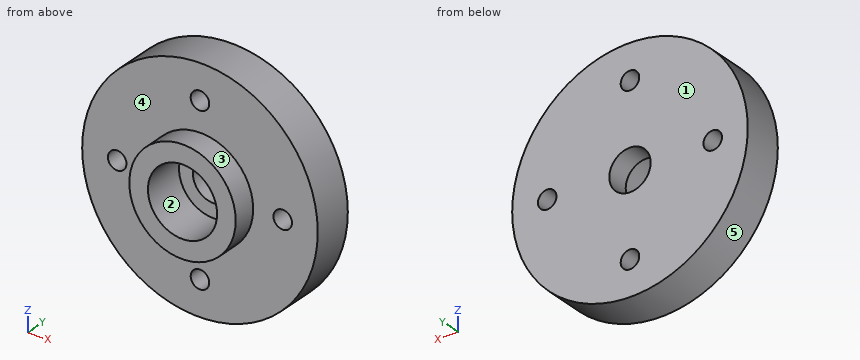
Autodesk Inventor part; units mm, degrees
ref_plane "YZ Plane" through (0, 0, 0) normal (1, 0, 0) x (0, 1, 0)
ref_plane "XZ Plane" through (0, 0, 0) normal (0, 1, 0) x (-1, 0, 0)
ref_plane "XY Plane" through (0, 0, 0) normal (0, 0, 1) x (1, 0, 0)
sketch "스케치1" plane through (0, 0, 0) normal (0, 0, 1) x (1, 0, 0)
  line L0 (0, 3.2752) -> (0, -3.2752)
  line L1 (1.75, 3.48) -> (1.75, 1.58)
  line L2 (1.75, 1.58) -> (2.925, 1.58)
  line L3 (2.925, 1.58) -> (2.925, -2.02)
  line L4 (2.925, -2.02) -> (4.5, -2.02)
  line L5 (4.5, -2.02) -> (4.5, 0)
  line L6 (4.5, 0) -> (9.96, 0)
  line L7 (9.96, 0) -> (9.96, 3.48)
  line L8 (9.96, 3.48) -> (1.75, 3.48)
  point P0 (0, 0)
  point P1 (0, 0)
  dimension "d1" = 1.75
  dimension "d2" = 2.925
  dimension "d4" = 3.48
  dimension "d6" = 4.5
  dimension "d7" = 9.96
  dimension "d8" = 1.9
  dimension "d22" = 5.5
revolve "회전1" add sketch "스케치1" angle 360 about axis through (0, 3.2752, 0) along (0, -1, 0)
sketch "Sketch3" plane through (0, 3.48, 0) normal (0, 1, 0) x (1, 0, 0)
  point P0 (0, 0)
  point P1 (7, 0)
  point P2 (0, 7)
  point P3 (-7, 0)
  point P4 (0, -7)
  dimension "d23" = 7
  dimension "d26" = 360
hole "Hole2" at (7, 3.48, 0) at (0, 3.48, -7) at (-7, 3.48, 0) at (0, 3.48, 7) direction (0, -1, 0) diameter 1.567 end through all
properties part number "Top Horn Metal" material "Aluminum 6061-AHC"
Work out the finished part from the listing and answer in its coordinate system (mm). Face numbers are marked on the shaded views. A direction names the side the tool comes from. Give positions to 0.01 mm unless a question says otherwise; leave off trailing zeros. Write each loop counter-clockwise with the first axis right and the second up, starting at its lowest first coordinate (ties: lowest second). Pieces come first, ordered by that corner, then holes.
Q1. The part is cut by section A-A on x = 0. State how many separate pieces and enclosed holes the cut face has, and give its area (3 significant figures).
Answer:
separate pieces: 4
enclosed holes: 0
area: 48.9 mm2
Q2. For a pull along X with two mould halves and no side action, classify the marked faces 1, 2 and 3 as released by +X, released by -X, zero draft, split by the parting line, or undercut.
Answer:
face 1: zero draft
face 2: undercut
face 3: split by the parting line
Q3. Given pin 1 (3 mm diameter, centred on x = 0, z = 0, fed in from +Y); pin 2 (1 mm diameter, centred on y = 0, z = 0.5, fed in from +X); pin 3 (3 mm diameter, centred on x = -5.5, z = -6.5, fed in from -Y); pin 4 (5.5 mm diameter, centred on x = 0, z = 0, fed in from -Y), each flat-ended and moving along its own axis, determine where each tip first touches the part or whether it passes through.
Answer:
pin 1: passes through
pin 2: stops at x = 9.96
pin 3: stops at y = 0
pin 4: stops at y = 1.58
Q4. A tool of negligible diameter and unlimited length cuts with its end or side. For the marked faces 4 and 5, from which of +Z, -Z, +X, -X, +Y, -Y can it reach the whole face along a straight path? Write none if from no direction.
Answer:
face 4: -Y
face 5: +Y, -Y
Q5. The part is cut by section D-D on x = -7. Give the vertices of the cut face in (y, z).
Answer:
outline: (0, -7.09) - (3.48, -7.09) - (3.48, -0.78) - (0, -0.78) - close; (0, 0.78) - (3.48, 0.78) - (3.48, 7.09) - (0, 7.09) - close
Q6. The part is cut by section C-C on z = -6.5. Give the vertices of the cut face in (x, y).
Answer:
outline: (-7.55, 0) - (-0.6, 0) - (-0.6, 3.48) - (-7.55, 3.48) - close; (0.6, 0) - (7.55, 0) - (7.55, 3.48) - (0.6, 3.48) - close
Q7. Straight lines are drawn through the part: L1, parallel to Z at x = 0, y = 2.4; L2, parallel to Z at x = 0.5, y = 1; L3, parallel to Y at x = 6.75, z = -2.75. For each, find the intervals that lie inside material, in ascending order.
Answer:
L1: z = -9.96 to -7.78, -6.22 to -1.75, 1.75 to 6.22, 7.78 to 9.96
L2: z = -9.95 to -7.6, -6.4 to -2.88, 2.88 to 6.4, 7.6 to 9.95
L3: y = 0 to 3.48
